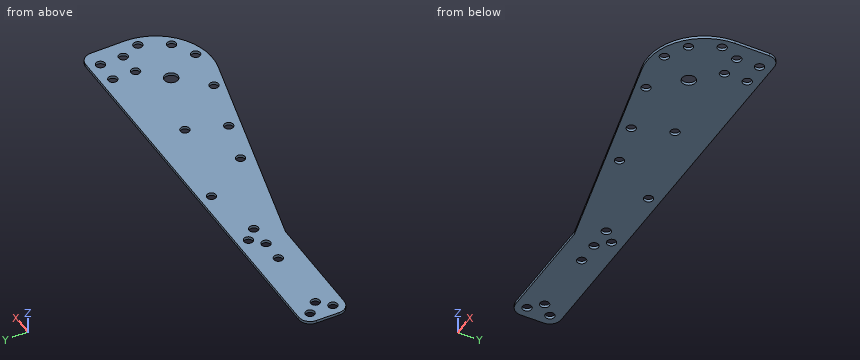
Autodesk Inventor part; units mm, degrees
ref_plane "YZ Plane" through (0, 0, 0) normal (1, 0, 0) x (0, 1, 0)
ref_plane "XZ Plane" through (0, 0, 0) normal (0, 1, 0) x (-1, 0, 0)
ref_plane "XY Plane" through (0, 0, 0) normal (0, 0, 1) x (1, 0, 0)
sketch "Sketch1" plane through (0, 0, 0) normal (0, 0, 1) x (1, 0, 0)
  line L0 (0, 0) -> (247.65, 0)
  line L1 (247.65, 0) -> (247.65, 38.1)
  line L2 (247.65, 38.1) -> (0, 38.1)
  line L3 (0, 38.1) -> (0, 0)
  line L4 (286.1616, 0) -> (255.1962, 0)
  line L5 (255.1962, 0) -> (255.1962, 12.7)
  line L6 (255.1962, 12.7) -> (286.1616, 12.7)
  line L7 (286.1616, 12.7) -> (286.1616, 0)
  line L8 (247.65, 12.7) -> (200.66, 12.7)
  line L9 (16.2468, 38.1) -> (16.2468, 12.7)
  line L10 (16.2468, 12.7) -> (196.85, 12.7)
  line L11 (0, 12.7) -> (17.7951, 12.7)
  circle A0 centre (200.66, 12.7) radius 31.75
  line L12 (232.41, 12.7) -> (231.9451, 38.1)
  line L13 (66.8614, 12.7) -> (200.8653, -20.0324)
  line L14 (193.3963, -18.208) -> (168.91, 12.7)
  point P0 (187.853, -16.3524)
  point P1 (232.3887, 13.8619)
  point P2 (229.7594, 0)
  point P3 (181.61, 38.1)
  point P4 (219.71, 38.1)
  point P5 (171.5606, 0)
  dimension "d0" = 247.65
  dimension "d1" = 38.1
  dimension "d2" = 12.7
  dimension "d3" = 30.9654
  dimension "d4" = 46.99
  dimension "d10" = 25.4
  dimension "d54" = 63.5
extrude "Extrusion4" add sketch "Sketch1" along normal blind 1.5875 contours L13 L0 A0 | L13 L10 A0 L0 | L3 L2 L9 L11 | A0 L14 L0 | L0 L14 A0 | L10 L9 L2 A0 | L14 L0 A0 | L14 A0 L2 L12 L0 | L2 L12 A0
fillet "Fillet6" radius 6.35 3 edges at (0, 38.1, 0.7937) (0, 12.7, 0.7937) (231.9451, 38.1, 0.7937)
sketch "Sketch4" plane through (0, 0, 1.5875) normal (0, 0, 1) x (1, 0, 0)
  arc A0 (6.35, 38.1) -> (0, 31.75) centre (6.35, 31.75) ccw
  line L0 (6.35, 38.1) -> (6.35, 31.75)
  line L1 (6.35, 31.75) -> (0, 31.75)
  circle A1 centre (6.35, 31.75) radius 2.54
  line L2 (6.35, 31.75) -> (6.35, 19.05)
  circle A2 centre (6.35, 19.05) radius 2.54
  line L3 (6.35, 31.75) -> (57.15, 31.75)
  line L4 (57.15, 31.75) -> (107.95, 31.75)
  line L5 (107.95, 31.75) -> (158.75, 31.75)
  line L6 (158.75, 31.75) -> (209.55, 31.75)
  circle A3 centre (107.95, 31.75) radius 2.54
  circle A4 centre (209.55, 31.75) radius 2.54
  line L7 (57.15, 31.75) -> (57.15, 19.05)
  line L8 (57.15, 19.05) -> (107.95, 19.05)
  line L9 (107.95, 19.05) -> (158.75, 19.05)
  line L10 (158.75, 19.05) -> (209.55, 19.05)
  circle A5 centre (158.75, 19.05) radius 2.54
  circle A6 centre (209.55, 19.05) radius 2.54
  line L11 (225.7103, 38.1) -> (6.35, 38.1)
  arc A7 (193.3963, -18.208) -> (232.41, 12.7) centre (200.66, 12.7) ccw
  line L12 (209.55, 31.75) -> (196.85, 31.75)
  line L13 (196.85, 31.75) -> (196.85, 19.05)
  circle A8 centre (196.85, 31.75) radius 2.54
  line L14 (196.85, 19.05) -> (196.85, 6.096)
  circle A9 centre (196.85, 6.096) radius 3.81
  line L15 (57.15, 31.75) -> (69.85, 31.75)
  circle A10 centre (69.85, 31.75) radius 2.54
  point P0 (0, 0)
  point P1 (207.01, 31.75)
  dimension "d60" = 6.35
  dimension "d61" = 5.08
  dimension "d62" = 12.7
  dimension "d63" = 5.08
  dimension "d64" = 50.8
  dimension "d65" = 50.8
  dimension "d66" = 50.8
  dimension "d67" = 50.8
  dimension "d70" = 5.08
  dimension "d72" = 5.08
  dimension "d75" = 5.08
  dimension "d76" = 5.08
  dimension "d86" = 12.7
  dimension "d88" = 5.08
  dimension "d89" = 12.954
  dimension "d90" = 7.62
  dimension "d116" = 12.7
  dimension "d117" = 5.08
extrude "Extrusion5" cut sketch "Sketch4" against normal blind 25.4 contours A4 | A6 | A9 | A2 | A1 L3 L0 | L0 L1 A1 | L1 L2 A1 | L3 A1 L2 | A10 L4 | L4 A10 | A3 L5 L4 | L4 L5 A3 | A5 L10 L9 | L9 L10 A5
sketch "Sketch5" plane through (0, 0, 1.5875) normal (0, 0, 1) x (1, 0, 0)
  circle A0 centre (209.55, 31.75) radius 2.54
  line L0 (209.55, 31.75) -> (222.25, 31.75)
  line L1 (222.25, 31.75) -> (222.25, 19.05)
  line L2 (222.25, 19.05) -> (226.6625, 8.5061)
  line L3 (226.6625, 8.5061) -> (219.2036, -6.223)
  line L4 (219.2036, -6.223) -> (207.01, -13.0403)
  line L5 (207.01, -13.0403) -> (181.8398, -9.6316)
  line L6 (181.8398, -9.6316) -> (151.2071, -1.2828)
  line L7 (151.2071, -1.2828) -> (126.701, 5.3962)
  circle A1 centre (126.701, 5.3962) radius 2.54
  circle A2 centre (151.2071, -1.2828) radius 2.54
  circle A3 centre (181.8398, -9.6316) radius 2.54
  circle A4 centre (207.01, -13.0403) radius 2.54
  circle A5 centre (219.2036, -6.223) radius 2.54
  circle A6 centre (226.6625, 8.5061) radius 2.54
  circle A7 centre (222.25, 19.05) radius 2.54
  circle A8 centre (222.25, 31.75) radius 2.54
  circle A9 centre (6.35, 19.05) radius 2.54
  line L8 (6.35, 19.05) -> (15.3303, 28.0303)
  line L9 (6.35, 19.05) -> (19.05, 19.05) construction
  circle A10 centre (6.35, 31.75) radius 2.54
  line L10 (6.35, 31.75) -> (15.3303, 22.7697)
  line L11 (6.35, 31.75) -> (19.05, 31.75) construction
  circle A11 centre (12.7, 25.4) radius 2.54
  line L12 (12.7, 25.4) -> (50.8, 25.4)
  circle A12 centre (50.8, 25.4) radius 2.54
  line L13 (12.7, 25.4) -> (25.4, 25.4)
  line L14 (25.4, 25.4) -> (38.1, 25.4)
  line L15 (50.8, 25.4) -> (63.5, 25.4)
  line L16 (63.5, 25.4) -> (76.2, 25.4)
  circle A13 centre (63.5, 25.4) radius 2.54
  circle A14 centre (76.2, 25.4) radius 2.54
  point P0 (0, 0)
  dimension "d91" = 12.7
  dimension "d92" = 12.7
  dimension "d93" = 11.43
  dimension "d94" = 16.51
  dimension "d95" = 13.97
  dimension "d96" = 25.4
  dimension "d97" = 31.75
  dimension "d98" = 25.4
  dimension "d99" = 5.08
  dimension "d100" = 5.08
  dimension "d101" = 5.08
  dimension "d102" = 5.08
  dimension "d103" = 5.08
  dimension "d104" = 5.08
  dimension "d105" = 5.08
  dimension "d106" = 5.08
  dimension "d109" = 12.7
  dimension "d110" = 45
  dimension "d111" = 12.7
  dimension "d112" = 45
  dimension "d113" = 5.08
  dimension "d114" = 38.1
  dimension "d115" = 5.08
  dimension "d118" = 12.7
  dimension "d119" = 12.7
  dimension "d122" = 12.7
  dimension "d123" = 12.7
  dimension "d124" = 5.08
  dimension "d125" = 5.08
extrude "Extrusion6" cut sketch "Sketch5" against normal blind 25.4 contours A1 | A2 L7 L6 | L6 L7 A2 | A3 L6 L5 | L5 L6 A3 | A4 L5 L4 | L4 L5 A4 | A5 L4 L3 | L3 L4 A5 | A6 L3 L2 | L2 L3 A6 | A7 L2 L1 | L1 L2 A7 | A8 L1 L0 | L0 L1 A8 | A14 | A13 L16 L15 | L15 L16 A13 | A12 L15 L12 | L12 L15 A12 | A11 L10 L8 | L8 L10 A11 | L10 A11 L8 | L12 A11 L10 | L8 A11 L12
fillet "Fillet7" radius 3.175 1 edges at (66.8614, 12.7, 0.7937)
properties part number "intake sled v5"
Input: part model. Units: mm. Frame: model coordinates. Coordinates: 2 decimals unless noted, no trailing zeros. Loops run counter-clockwise (first coordinate to the right, second up) from the corner with the lowest first, then second, coordinate; pieces in that order, holes last. Notation, with made-up numbers: (30.25, 72) - (64.25, 72) arc R14 cw to (64.25, 89) - close; hole circle Ø6 at (31.5, 29.5). An arc over 180 degrees is marked (long way). Answer in a Markdown table with one row per item. Add a question column.
Item 1: Contact query for a flat-ended pin moving along its axis: P1, Ø3, axis at x = 6.35, y = 19.05, coming from the -Z side. Output: stop coordinate, or through.
Item 2: Section query A-A on x = 158.75. Return the cut outline in (y, z).
Item 3: Section query D-D on x = 28. Return the cut outline in (y, z).
Item 4: Section query C-C on x = 63.5. Return the cut outline in (y, z), then the cut area to 3 significant figures.
Item 5: Line query: line 1 along X through (y, z) = (31.75, 1.15); line 2 along X through (y, z) = (19.05, 0.5); line 3 along X through (y, z) = (24, 0.3). Output: solid intervals per line, ascending. Write a range as [from, to].
Item 6: Section query B-B on z = 0.65. State how many separate pieces and enclosed holes the cut face has, then the cut area to 3 significant figures.
Recorded:
| question | item | result |
|---|---|---|
| 1 | P1 | through |
| 2 | outline | (-9.75, 0) - (16.51, 0) - (16.51, 1.59) - (-9.75, 1.59) - close; (21.59, 0) - (38.1, 0) - (38.1, 1.59) - (21.59, 1.59) - close |
| 3 | outline | (12.7, 0) - (38.1, 0) - (38.1, 1.59) - (12.7, 1.59) - close |
| 4 | outline | (12.7, 0) - (22.86, 0) - (22.86, 1.59) - (12.7, 1.59) - close; (27.94, 0) - (38.1, 0) - (38.1, 1.59) - (27.94, 1.59) - close |
| 4 | area | 32.3 mm^2 |
| 5 | line 1 | [0, 3.81], [8.89, 67.31], [72.39, 105.41], [110.49, 207.01], [212.09, 219.71], [224.79, 232.06] |
| 5 | line 2 | [0, 3.81], [8.89, 156.21], [161.29, 207.01], [212.09, 219.71], [224.79, 232.29] |
| 5 | line 3 | [0, 10.58], [14.82, 48.68], [52.92, 61.38], [65.62, 74.08], [78.32, 232.2] |
| 6 | separate pieces | 1 |
| 6 | enclosed holes | 20 |
| 6 | area | 8,420 mm^2 |
